```python
from build123d import *

# Parameters (mm, degrees)
F0_R     = 4.55
F1_DEPTH = 5.5
F2_R     = 2.5
F3_DEPTH = 20
F5_DEPTH = 2.5
F6_SIZE2 = 0.5773502692
F6_SIZE  = 1
F7_SIZE  = 0.8


with BuildPart() as f1:
    # F0 (on Top) → F1 (new body)
    with BuildSketch(Plane.XY):
        Circle(F0_R)
    extrude(amount=-F1_DEPTH)

    # F2 (on face) → F3 (join)
    with BuildSketch(Plane(origin=(0, 0, -5.5), x_dir=(1, 0, 0), z_dir=(0, 0, -1))):
        Circle(F2_R)
    extrude(amount=F3_DEPTH)

    # F4 (on face) → F5 (cut)
    with BuildSketch(Plane.XY):
        Polygon((-0.0040677853, -2.3093974943), (1.9979630048, -1.1582215525), (2.0020307901, 1.1511759417), (0.0040677853, 2.3093974943), (-1.9979630048, 1.1582215525), (-2.0020307901, -1.1511759417), align=None)
    extrude(amount=-F5_DEPTH, mode=Mode.SUBTRACT)

    # F6
    f6_edges = [f1.edges().sort_by_distance(p)[0] for p in [
        (-4.55, 0, 0),
    ]]
    f6_side = f1.faces().sort_by_distance((-4.421307, 0, 0))[0]
    chamfer(f6_edges, length=F6_SIZE, length2=F6_SIZE2, reference=f6_side)

    # F7
    f7_edges = [f1.edges().sort_by_distance(p)[0] for p in [
        (-2.5, 0, -25.5),
    ]]
    chamfer(f7_edges, length=F7_SIZE)


solid = f1.part
```
Work out the finished part from the listing and answer in its coordinate system (mm). A direction names the side the tool comes from. Give positions to 0.01 mm unless a question says otherwise; leave off trailing zeros. Write each loop counter-clockwise with the first axis right and the second up, starting at its lowest first coordinate (ties: lowest second). Pieces come first, ordered by that corner, then holes. Notation, with made-up numbers: (71.5, 32.25) -> (109.5, 32.25) arc R24 ccw to (109.5, 60.25) -> close; hole circle Ø2 at (29, 83.25). An arc over 180 degrees is marked (long way). Write item = value, one per line.
Q1. For a pull along X with two mould halves and no side action, classify faces 1 (the flat face through (2, -2, -5.5)), 2 (the flat face through (0.983, -1.742, -1.232)), 3 (the cylindrical face through (-0.99, -4.44, -3)) as pulls with the +X half, pulls with the -X half, needs draft (parallel to the pull), parting line crosses it, or undercut.
Computed values:
face_1 = needs draft
face_2 = undercut
face_3 = parting line crosses it
Q2. A tool of negligible diameter and unlimited length cuts with its end or side. For faces 4 (the flat face through (2, -2, 0)), 5 (the flat face through (-0.983, 1.742, -1.232)), 6 (the cylindrical face through (-0.54, 2.44, -14.97)), from which of +Z, -Z, +X, -X, +Y, -Y can it reach the whole face along a straight path? Write none if from no direction.
Computed values:
face_4 = +Z, +X, -X, +Y, -Y
face_5 = +Z
face_6 = -Z
Q3. Flat-ended cylindrical pins translate along their axes: pin 1 Ø4 at (x, z) = (0, -16.5) entering from -Y; pin 2 Ø1.2 at (x, y) = (0, 0.5) entering from +Z; pin 3 Ø3 at (y, z) = (-2.5, -15.5) entering from +X. Find the tip coordinate at first contact, or state that the pin passes through.
Computed values:
pin_1 = -2.5
pin_2 = -2.5
pin_3 = 2.29
Q4. Section A-A on z = -4.5 is taken. Determine the outline of the cut face in (x, y), and give its area (3 significant figures).
Computed values:
outline = circle Ø9.1 at (0, 0)
area = 65.0 mm^2
Q5. Section B-B on z = -20 is taken. Determine the outline of the cut face in (x, y).
Computed values:
outline = circle Ø5 at (0, 0)
Q6. Consider line 1 along Z through (x, y) = (1, 2.75); line 2 along X through (y, z) = (2.25, -2); line 3 along Z through (x, y) = (-1, 1.25). Determine where each line is inside the solid, lowest interval first.
Computed values:
line_1 = -5.5 to 0
line_2 = -3.95 to -0.1, 0.11 to 3.95
line_3 = -25.5 to -2.5
